Work out the finished part from the listing and answer in its coordinate system (mm). Round coordinates to 2 decimals unless told otherwise and drop trailing zeros. Write each loop counter-clockwise with the first axis right and the second up, starting at its lowest first coordinate (ties: lowest second). Pieces come first, ordered by that corner, then holes. Notation, with made-up numbers: M -29,84.25 L 15,84.25 A21 ccw 15,110.25 Z; hole C 31,-5.75 d4. An arc over 180 degrees is marked long. Answer in a Markdown table with one row per item.
```python
from build123d import *

# Parameters (mm, degrees)
F2_R          = 12.7
F6_DEPTH      = 19.05
F6_DEPTH_BACK = 430.53
F8_R          = 3.175
F9_DEPTH      = 19.05
F9_DEPTH_BACK = 425.958
F10_R         = 2.54


with BuildPart() as f3:
    # F3: sweep along a path in F1
    with BuildLine(Plane.XY) as f3_path:
        Line((-203.2, -101.6), (-203.2, 0))
        Line((-203.2, 0), (-203.2, 228.6))
        ThreePointArc((-203.2, 228.6), (-180.8815367264, 282.4815367264), (-127, 304.8))
        Line((-127, 304.8), (0, 304.8))
        Line((0, 304.8), (127, 304.8))
        ThreePointArc((127, 304.8), (180.8815367264, 282.4815367264), (203.2, 228.6))
        Line((203.2, 228.6), (203.2, 0))
    # F2 (on offset) → F3 (sweep)
    with BuildSketch(Plane.XZ.offset(101.6)):
        with Locations((-203.2, 0)):
            Circle(F2_R)
    sweep(path=f3_path.line)

    # F5 (on offset) → F6 (cut, two sides)
    with BuildSketch(Plane.YZ.offset(203.2)) as f6_sk:
        with BuildLine():
            ThreePointArc((200.025, 0), (203.2, -3.175), (206.375, 0))
            ThreePointArc((206.375, 0), (203.2, 3.175), (200.025, 0))
        make_face()
    extrude(amount=F6_DEPTH, mode=Mode.SUBTRACT)
    extrude(f6_sk.sketch, amount=-F6_DEPTH_BACK, mode=Mode.SUBTRACT)

    # F7: F3 across plane


with BuildPart() as f3_1:
    add(f3.part)
    add(f3.part.mirror(Plane.YZ))

    # F8 (on offset) → F9 (cut, two sides)
    with BuildSketch(Plane.YZ.offset(203.2)) as f9_sk:
        with Locations((-76.2, 0)):
            Circle(F8_R)
    extrude(amount=F9_DEPTH, mode=Mode.SUBTRACT)
    extrude(f9_sk.sketch, amount=-F9_DEPTH_BACK, mode=Mode.SUBTRACT)

    # F10
    f10_edges = [f3_1.edges().sort_by_distance(p)[0] for p in [
        (-215.9, -101.6, 0),
        (215.9, -101.6, 0),
    ]]
    fillet(f10_edges, radius=F10_R)


solid = f3_1.part
```
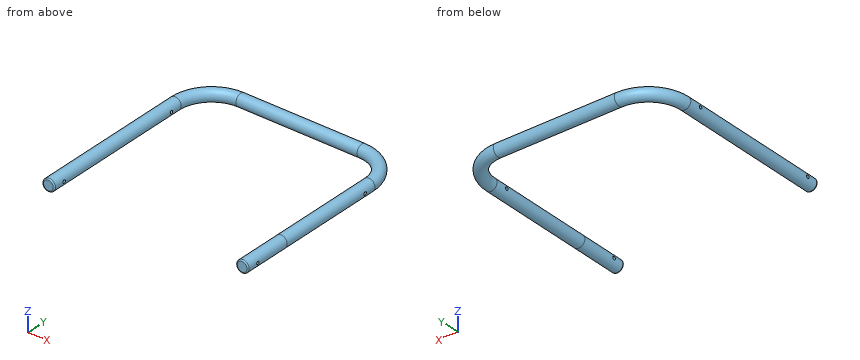
1. Given pin 1 (1 mm diameter, centred on y = -17.5, z = -4, fed in from +X); pin 2 (1 mm diameter, centred on x = -81.5, z = -4, fed in from +Y); pin 3 (2 mm diameter, centred on x = -14.5, z = -5, fed in from -Y), each flat-ended and moving along its own axis, determine where each tip first touches the part or whether it passes through.
Calculated:
| item | result |
|---|---|
| pin 1 | stops at x = 215.41 |
| pin 2 | stops at y = 317.01 |
| pin 3 | stops at y = 292.75 |
2. The part is cut by section B-B (x = -203.2). Count the separate pieces of the cut face and the enclosed holes in it, plus the area to 3 significant figures.
Calculated:
| item | result |
|---|---|
| separate pieces | 1 |
| enclosed holes | 2 |
| area | 9,330 mm² |
3. The part is cut by section C-C (x = -24). Determine the outline of the cut face in (y, z), plus the area to 3 significant figures.
Calculated:
| item | result |
|---|---|
| outline | C 304.8,0 d25.4 |
| area | 507 mm² |
4. The part is cut by section A-A (y = 155.5). Determine the outline of the cut face in (x, z), plus the area to 3 significant figures.
Calculated:
| item | result |
|---|---|
| outline | C -203.2,0 d25.4; C 203.2,0 d25.4 |
| area | 1,010 mm² |
5. Consider line 1 along Z through (x, y) = (-204, 203); line 2 along Y through (x, z) = (-195.75, 0) (3 decimals); line 3 along Y through (x, z) = (-196.25, 0) (3 decimals). Determine where each line is inside the solid, lowest interval first. Write a range as from..to.
Calculated:
| item | result |
|---|---|
| line 1 | z = -12.67..-3.17, 3.17..12.67 |
| line 2 | y = -101.6..-79.375, -73.025..200.025, 206.375..284.962 |
| line 3 | y = -101.6..-79.375, -73.025..200.025, 206.375..284.346 |
